The model under review builds one solid part; all positions refer to its coordinate system, in mm. Face numbers are marked on the shaded views. Coordinates: 2 decimals unless noted, no trailing zeros. Order: outer loops, then holes, each group sorted by start corner. A loop starts at its lowest first (then second) coordinate and runs counter-clockwise, first axis right, second up.
```python
from build123d import *

# Parameters (mm, degrees)
SKETCH1_W      = 203.2
SKETCH1_H      = 101.6
EXTRUDE1_DEPTH = 50.8
EXTRUDE2_DEPTH = 16.51
SKETCH22_W     = 203.2
SKETCH22_H     = 50.8
EXTRUDE3_DEPTH = 12700


with BuildPart() as part:
    # Sketch1 → Extrude1 (new body)
    with BuildSketch(Plane.XY):
        with Locations((101.6, 50.8)):
            Rectangle(SKETCH1_W, SKETCH1_H)
    extrude(amount=EXTRUDE1_DEPTH)

    # Sketch20 → Extrude2 (add)
    with BuildSketch(Plane.XY.offset(50.8)):
        with BuildLine():
            ThreePointArc((98.73765298, 90.37654578), (100.476619995, 89.229944151), (102.493050685, 88.707728828))
            Line((102.493050685, 88.707728828), (157.48, 83.82))
            Line((157.48, 83.82), (157.48, 78.74))
            Line((157.48, 78.74), (154.94, 78.74))
            Line((154.94, 78.74), (154.94, 74.422))
            Line((154.94, 74.422), (93.98, 74.422))
            Line((93.98, 74.422), (93.947422963, 78.74))
            Line((93.947422963, 78.74), (91.44, 78.74))
            Line((91.44, 78.74), (89.009960204, 84.606635031))
            Line((89.009960204, 84.606635031), (81.969998167, 81.690587277))
            Line((81.969998167, 81.690587277), (79.539958371, 87.557222308))
            Line((79.539958371, 87.557222308), (86.579920409, 90.473270063))
            Line((86.579920409, 90.473270063), (83.023180413, 99.06))
            Line((83.023180413, 99.06), (89.373180413, 99.06))
            Line((89.373180413, 99.06), (98.73765298, 90.37654578))
        make_face()
    extrude(amount=EXTRUDE2_DEPTH)

    # Sketch22 → Extrude3 (cut)
    with BuildSketch(Plane(origin=(0, 101.6, 0), x_dir=(1, 0, 0), z_dir=(0, 1, 0))):
        with Locations((101.6, -25.4)):
            Rectangle(SKETCH22_W, SKETCH22_H)
    extrude(amount=-EXTRUDE3_DEPTH, mode=Mode.SUBTRACT)


solid = part.part
```
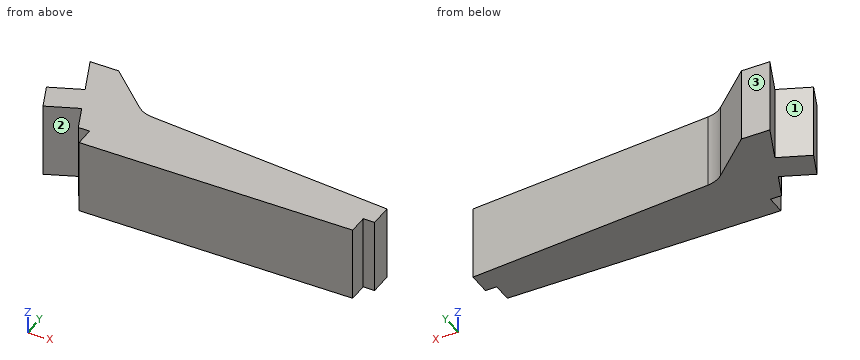
(1) For pin 1 Ø0.8 at (x, z) = (156.5, 55.5) entering from -Y; pin 2 Ø6 at (y, z) = (87.5, 57) entering from -X; pin 3 Ø4 at (y, z) = (96, 54.5) entering from +X, all flat-tipped, find the tip position at first contact; note any pin that passes through.
A:
pin 1: stops at y = 78.74
pin 2: stops at x = 79.54
pin 3: stops at x = 94.83
(2) We need section B-B, the plane y = 85.5. Write out the cut boundary in (x, z).
A:
outline: (80.39, 50.8) - (138.58, 50.8) - (138.58, 67.31) - (80.39, 67.31) - close
(3) We need section A-A, the plane z = 63. Write out the cut boundary in (x, y), and give its area (3 significant figures).
A:
outline: (79.54, 87.56) - (81.97, 81.69) - (89.01, 84.61) - (91.44, 78.74) - (93.95, 78.74) - (93.98, 74.42) - (154.94, 74.42) - (154.94, 78.74) - (157.48, 78.74) - (157.48, 83.82) - (102.49, 88.71) arc R6.35 cw to (98.74, 90.38) - (89.37, 99.06) - (83.02, 99.06) - (86.58, 90.47) - close
area: 958 mm2
(4) We need section C-C, the plane x = 122.5. Write out the cut boundary in (y, z), and give its area (3 significant figures).
A:
outline: (74.42, 50.8) - (86.93, 50.8) - (86.93, 67.31) - (74.42, 67.31) - close
area: 206 mm2
(5) Draft analysis for pull direction X (two halves, no side actions). For the marked faces 1, 2 and 3, state which applies: released by +X, released by -X, zero draft, split by the parting line, or undercut.
A:
face 1: released by -X
face 2: undercut
face 3: zero draft
(6) Wall thickness on probe 1 along X at (y, z) = (78.5, 65); probe 2 along X at (y, z) = (76, 52.75); probe 3 along Y at (x, z) = (133.5, 56.25): over which ranges is each line inside the solid? List them lowest first.
A:
probe 1: x = 93.95 to 154.94
probe 2: x = 93.97 to 154.94
probe 3: y = 74.42 to 85.95
